```python
from build123d import *

# Parameters (mm, degrees)
SKETCH008_R           = 43
SKETCH008_R_2         = 4
PAD002_DEPTH          = 12
SKETCH009_R           = 11
POCKET002_DEPTH       = 7
SKETCH010_R           = 3
POCKET003_DEPTH       = 256.426858
POLARPATTERN001_COUNT = 6
SKETCH011_R           = 2.75
POCKET004_DEPTH       = 256.426858
POLARPATTERN002_COUNT = 8


with BuildPart() as part:
    # Sketch008 (on Face1 of ShapeBinder003) → Pad002 (new body)
    with BuildSketch(Plane.XZ.offset(8)):
        Circle(SKETCH008_R)
        Circle(SKETCH008_R_2, mode=Mode.SUBTRACT)
    extrude(amount=PAD002_DEPTH)

    # Sketch009 (on Face3 of Pad002) → Pocket002 (cut)
    with BuildSketch(Plane(origin=(0, -8, 0), x_dir=(1, 0, 0), z_dir=(0, 1, 0))):
        Circle(SKETCH009_R)
    extrude(amount=-POCKET002_DEPTH, mode=Mode.SUBTRACT)

    # Sketch010 (on Face2 of Pocket002) → Pocket003 (cut, through all)
    with BuildSketch(Plane(origin=(0, -8, 0), x_dir=(1, 0, 0), z_dir=(0, 1, 0))):
        with Locations((0, 16)):
            Circle(SKETCH010_R)
    pocket003 = extrude(amount=-POCKET003_DEPTH, mode=Mode.SUBTRACT)

    # PolarPattern001: Pocket003 ×6 about axis
    polarpattern001_axis = Axis((0, -8, 0), (0, 1, 0))
    for i in range(1, POLARPATTERN001_COUNT):
        add(pocket003.rotate(polarpattern001_axis, i * 360 / POLARPATTERN001_COUNT), mode=Mode.SUBTRACT)

    # Sketch011 (on Face2 of PolarPattern001) → Pocket004 (cut, through all)
    with BuildSketch(Plane(origin=(0, -8, 0), x_dir=(1, 0, 0), z_dir=(0, 1, 0))):
        with Locations((0, 38)):
            Circle(SKETCH011_R)
    pocket004 = extrude(amount=-POCKET004_DEPTH, mode=Mode.SUBTRACT)

    # PolarPattern002: Pocket004 ×8 about axis
    polarpattern002_axis = Axis((0, -8, 0), (0, 1, 0))
    for i in range(1, POLARPATTERN002_COUNT):
        add(pocket004.rotate(polarpattern002_axis, i * 360 / POLARPATTERN002_COUNT), mode=Mode.SUBTRACT)


solid = part.part
```
Input: part model. Units: mm. Frame: model coordinates. A direction names the side the tool comes from. Coordinates: 2 decimals unless noted, no trailing zeros. Write each loop counter-clockwise with the first axis right and the second up, starting at its lowest first coordinate (ties: lowest second). Pieces come first, ordered by that corner, then holes.
1) Section A-A on z = 0. Output: boundary loops of the cut face in (x, y).
2) Section C-C on z = -27. Output: boundary loops of the cut face in (x, y), and give its area (3 significant figures).
3) Material intervals for line 1 along Z through (x, y) = (26, -14); line 2 along Z through (x, y) = (0, -17.9); line 3 along X through (y, z) = (-10.5, -25), sorted ascending.
4) Section B-B on x = 38. Output: boundary loops of the cut face in (y, z), and give its area (3 significant figures).
5) Mould query, pull axis X, two halves, no side actions, for faces 3 (the cylindrical face through (-2.38, -11.45, 10.74)), 4 (the cylindrical face through (-10.995, -13.916, 7.099)), 5 (the cylindrical face through (-5.598, -13.916, 42.634)), 6 (the flat face through (9, -20, 1)). Classes: pulls with the +X half, pulls with the -X half, needs draft (parallel to the pull), parting line crosses it, or undercut.
6) Section D-D on y = -11.75. State how many separate pieces and enclosed holes the cut face has, and give its area (3 significant figures).
7) Pin query (flat end, axial travel): pin 1 Ø6.5 at (x, z) = (26.87, -26.87) entering from -Y; pin 2 Ø1 at (x, y) = (19.5, -16.5) entering from +Z; pin 3 Ø2 at (y, z) = (-18.5, -2) entering from +X; pin 4 Ø20 at (x, z) = (0, 0) entering from +Y. Return the tip coordinate at first contact, or that it passes through.
8) Set-up query: faces 1 (the flat face through (0, -15, 5)), 2 (the cylindrical face through (-0.358, -13.916, -40.727)). Return all of +Z, -Z, +X, -X, +Y, -Y with unobstructed straight access to the full face (end or side cutting, diameter ignored); none if empty.
Check result:
1. outline: (-43, -20) - (-40.75, -20) - (-40.75, -8) - (-43, -8) - close; (-35.25, -20) - (-4, -20) - (-4, -15) - (-11, -15) - (-11, -8) - (-35.25, -8) - close; (4, -20) - (35.25, -20) - (35.25, -8) - (11, -8) - (11, -15) - (4, -15) - close; (40.75, -20) - (43, -20) - (43, -8) - (40.75, -8) - close
2. outline: (-33.47, -20) - (-29.62, -20) - (-29.62, -8) - (-33.47, -8) - close; (-24.12, -20) - (24.12, -20) - (24.12, -8) - (-24.12, -8) - close; (29.62, -20) - (33.47, -20) - (33.47, -8) - (29.62, -8) - close
2. area: 671 mm2
3. line 1: z = -34.25 to -29.48, -24.26 to 24.26, 29.48 to 34.25
3. line 2: z = -43 to -40.75, -35.25 to -19, -13 to -4, 4 to 13, 19 to 35.25, 40.75 to 43
3. line 3: x = -34.99 to -28.89, -24.85 to 24.85, 28.89 to 34.99
4. outline: (-20, -20.12) - (-8, -20.12) - (-8, -2.75) - (-20, -2.75) - close; (-20, 2.75) - (-8, 2.75) - (-8, 20.12) - (-20, 20.12) - close
4. area: 417 mm2
5. face 3: undercut
5. face 4: undercut
5. face 5: parting line crosses it
5. face 6: needs draft
6. separate pieces: 1
6. enclosed holes: 15
6. area: 5,070 mm2
7. pin 1: stops at y = -20
7. pin 2: stops at z = 38.57
7. pin 3: stops at x = 42.99
7. pin 4: stops at y = -15
8. face 1: +Y
8. face 2: +Y, -Y
